Can you work these out from the model? Positions are in its coordinate system, mm. A direction names the side the tool comes from. Coordinates: 2 decimals unless noted, no trailing zeros. Loops run counter-clockwise (first coordinate to the right, second up) from the corner with the lowest first, then second, coordinate; pieces in that order, holes last. Notation, with made-up numbers: (-32.5, 72.5) -> (-15.5, 72.5) arc R14 cw to (-15.5, 97.5) -> close; hole circle Ø4 at (73.25, 50). An arc over 180 degrees is marked (long way). Use one line per item in the form item = value. Start each with the question number.
(1) On a 3-axis mill with a long thin cutter (end or side, diameter ignored), from which of +Z, -Z, +X, -X, +Y, -Y can I reach the whole of each face in a straight line? I mean faces 1 (the flat face through (-27.5, 23, 1)), 2 (the flat face through (27.5, 22, 1)), 3 (the flat face through (-31, 8, 1)). Say none if no direction works.
(2) Imagine slicing it at B-B (z = 0.95). State how many separate pieces and enclosed holes the cut face has, plus the area to 3 significant figures.
(3) I'm going to push flat-ended pins straight in: pin 1 (1.5 mm diameter, centred on x = 30, z = 1, fed in from -Y); pin 2 (2.5 mm diameter, centred on x = -27.5, y = 8, fed in from -Z); pin 3 (1.5 mm diameter, centred on y = 2, z = 2, fed in from +X). Where does each tip first touch, or does it pass through?
(4) Thinking about a two-plate mould opening in Y: for faces 4 (the cylindrical face through (10.73, 0.683, 1.521)), 5 (the flat face through (32.5, 13, 1)), 6 (the flat face through (0, 0, 1)), which applies, released by +Y, released by -Y, zero draft, split by the parting line, or undercut?
(5) I need wall thicknesses on line 1 (Y direction, x = 22.5, z = 1.8); line 2 (X direction, y = 6, z = 0.3); line 3 (X direction, y = 2, z = 2.75). Which ranges of each line are inside material? Lowest first, please. Write a range as [from, to].
(6) Imagine slicing it at A-A (y = 5). List the corners of the cut face in (x, z) for me.
```python
from build123d import *

# Parameters (mm, degrees)
EXTRUDE_1_OUTLINE_R = 1.45
EXTRUDE_1_DEPTH     = 3
SKETCH_2_R          = 1
CUT_EXTRUDE_1_DEPTH = 42.728287915
FILLET_1_R          = 3


# Read off the part's stored shape, not the designer's step: 凸台-拉伸1
with BuildPart() as part:
    # 凸台-拉伸1 outline → 凸台-拉伸1 (new body)
    with BuildSketch(Plane.XY):
        with BuildLine():
            Line((32.5, 8), (32.5, 18))
            Line((32.5, 18), (27.5, 18))
            Line((27.5, 18), (27.5, 26))
            Line((27.5, 26), (19.5, 26))
            add(Edge.make_bspline(
                [(19.5, 26), (19.5, 10), (-19.5, 10), (-19.5, 26)],
                knots=[0, 0, 0, 1, 2, 2, 2], degree=2))
            Line((-19.5, 26), (-27.5, 26))
            Line((-27.5, 26), (-27.5, 18))
            Line((-27.5, 18), (-32.5, 18))
            Line((-32.5, 18), (-32.5, 8))
            Line((-32.5, 8), (-27.5, 8))
            Line((-27.5, 8), (-27.5, 0))
            Line((-27.5, 0), (-20, 0))
            Line((-20, 0), (-20, -5))
            Line((-20, -5), (-10, -5))
            Line((-10, -5), (-10, 0))
            Line((-10, 0), (10, 0))
            Line((10, 0), (10, -5))
            Line((10, -5), (20, -5))
            Line((20, -5), (20, 0))
            Line((20, 0), (27.5, 0))
            Line((27.5, 0), (27.5, 8))
            Line((27.5, 8), (32.5, 8))
        make_face()
        with Locations((-22.5, 5)):
            Circle(EXTRUDE_1_OUTLINE_R, mode=Mode.SUBTRACT)
        with Locations((22.5, 5)):
            Circle(EXTRUDE_1_OUTLINE_R, mode=Mode.SUBTRACT)
    extrude(amount=EXTRUDE_1_DEPTH)

    # 草图2 → 切除-拉伸1 (cut, through all)
    with BuildSketch(Plane.XY.offset(3)):
        with Locations((-27.5, 18)):
            Circle(SKETCH_2_R)
        with Locations((-27.5, 8)):
            Circle(SKETCH_2_R)
        with Locations((-20, 0)):
            Circle(SKETCH_2_R)
        with Locations((-10, 0)):
            Circle(SKETCH_2_R)
        with Locations((10, 0)):
            Circle(SKETCH_2_R)
        with Locations((20, 0)):
            Circle(SKETCH_2_R)
        with Locations((27.5, 8)):
            Circle(SKETCH_2_R)
        with Locations((27.5, 18)):
            Circle(SKETCH_2_R)
    extrude(amount=-CUT_EXTRUDE_1_DEPTH, mode=Mode.SUBTRACT)

    # 圆角1
    fillet_1_edges = [part.edges().sort_by_distance(p)[0] for p in [
        (19.5, 26, 1.5),
        (-19.5, 26, 1.5),
    ]]
    fillet(fillet_1_edges, radius=FILLET_1_R)


solid = part.part
```
Worked out:
q1.face_1 = +Z, -Z, -X, +Y
q1.face_2 = +Z, -Z, +X, +Y
q1.face_3 = +Z, -Z, -X, -Y
q2.separate_pieces = 1
q2.enclosed_holes = 2
q2.area = 1,070 mm2
q3.pin_1 = 8
q3.pin_2 = 0
q3.pin_3 = 27.5
q4.face_4 = undercut
q4.face_5 = zero draft
q4.face_6 = released by -Y
q5.line_1 = [0, 3.55], [6.45, 26]
q5.line_2 = [-27.5, -23.55], [-21.45, 21.45], [23.55, 27.5]
q5.line_3 = [-27.5, 27.5]
q6.outline = (-27.5, 0) -> (-23.95, 0) -> (-23.95, 3) -> (-27.5, 3) -> close; (-21.05, 0) -> (21.05, 0) -> (21.05, 3) -> (-21.05, 3) -> close; (23.95, 0) -> (27.5, 0) -> (27.5, 3) -> (23.95, 3) -> close
